Verification items for the finished model (mm, model axes). A direction names the side the tool comes from. Round coordinates to 2 decimals unless told otherwise and drop trailing zeros. Write each loop counter-clockwise with the first axis right and the second up, starting at its lowest first coordinate (ties: lowest second). Pieces come first, ordered by that corner, then holes.
Autodesk Fusion 360 part; units mm, degrees
sketch "Sketch1" plane through (0, 0, 0) normal (0, 1, 0) x (1, 0, 0)
  line L0 (0, 0) -> (49, 0)
  line L1 (49, 0) -> (49, -24)
  line L2 (49, -24) -> (0, -24)
  line L3 (0, -24) -> (0, 0)
extrude "Extrude1" add sketch "Sketch1" along normal blind 2
sketch "Sketch2" plane through (0, 0, 0) normal (0, 1, 0) x (1, 0, 0)
  line L0 (10, 0) -> (39, 0)
  line L1 (39, 0) -> (39, -14)
  line L2 (39, -14) -> (10, -14)
  line L3 (10, -14) -> (10, 0)
extrude "Extrude2" add sketch "Sketch2" against normal blind 5
fillet "Fillet1" radius 3 1 edges at (0, 1, 24)
fillet "Fillet2" radius 3 1 edges at (49, 1, 24)
fillet "Fillet3" radius 3 1 edges at (49, 1, 0)
fillet "Fillet4" radius 3 1 edges at (0, 1, 0)
sketch "Sketch3" plane through (0, 0, 0) normal (0, 1, 0) x (1, 0, 0)
  circle A0 centre (5, -5) radius 2.5
  dimension "d13" = 5
extrude "Extrude3" cut sketch "Sketch3" along normal blind 3
sketch "Sketch4" plane through (0, 0, 0) normal (0, 1, 0) x (1, 0, 0)
  circle A0 centre (44, -5) radius 2.5
  dimension "d16" = 5
extrude "Extrude4" cut sketch "Sketch4" along normal blind 3
sketch "Sketch5" plane through (0, 0, 0) normal (0, 1, 0) x (1, 0, 0)
  circle A0 centre (5, -19) radius 2.5
  dimension "d19" = 5
extrude "Extrude5" cut sketch "Sketch5" along normal blind 3
sketch "Sketch6" plane through (0, 0, 0) normal (0, 1, 0) x (1, 0, 0)
  circle A0 centre (44, -19) radius 2.5
  dimension "d22" = 5
extrude "Extrude6" cut sketch "Sketch6" along normal blind 3
sketch "Sketch7" plane through (0, 0, 0) normal (0, 1, 0) x (1, 0, 0)
  circle A0 centre (44, -12) radius 2.5
  dimension "d25" = 5
extrude "Extrude7" cut sketch "Sketch7" along normal blind 2
sketch "Sketch8" plane through (0, 0, 0) normal (0, 1, 0) x (1, 0, 0)
  circle A0 centre (5, -12) radius 2.5
  dimension "d28" = 5
extrude "Extrude8" cut sketch "Sketch8" along normal blind 3
sketch "Sketch9" plane through (0, 0, 0) normal (0, 1, 0) x (1, 0, 0)
  circle A0 centre (25, -19) radius 2.5
  dimension "d31" = 5
extrude "Extrude9" cut sketch "Sketch9" along normal blind 3
sketch "Sketch10" plane through (0, 0, 0) normal (0, 1, 0) x (1, 0, 0)
  circle A0 centre (15, -19) radius 2.5
  dimension "d34" = 5
extrude "Extrude10" cut sketch "Sketch10" along normal blind 2
sketch "Sketch11" plane through (0, 0, 0) normal (0, 1, 0) x (1, 0, 0)
  circle A0 centre (35, -19) radius 2.5
  dimension "d37" = 5
extrude "Extrude11" cut sketch "Sketch11" along normal blind 5
Q1. Release check for a two-part mould opening along Z. For faces 1 (the cylindrical face through (48.1, 1.01, 23.14)), 2 (the flat face through (24.2, 0, 14.5)), 3 (the cylindrical face through (6.34, 0.99, 21.11)) record: released by +Z, released by -Z, zero draft, split by the parting line, or undercut.
Recorded:
face 1: released by +Z
face 2: zero draft
face 3: undercut
Q2. Depth check by flat-ended pin: P1, Ø3, axis at x = 15, z = 19, coming from the -Y side; P2, Ø8, axis at x = 44, z = 5, coming from the -Y side; P3, Ø2.5, axis at x = 26.5, y = -2.5, coming from the +Z side; P4, Ø1.5, axis at y = -2.5, z = 8.5, coming from the -X side. Enter the tip coordinate at first touch or a pass-through.
Recorded:
P1: passes through
P2: stops at y = 0
P3: stops at z = 14
P4: stops at x = 10
Q3. Sectioned sample at D-D (z = 19). Enter the section's corners in (x, y), plus the area to 3 significant figures.
Recorded:
outline: (0, 0) - (2.5, 0) - (2.5, 2) - (0, 2) - close; (7.5, 0) - (12.5, 0) - (12.5, 2) - (7.5, 2) - close; (17.5, 0) - (22.5, 0) - (22.5, 2) - (17.5, 2) - close; (27.5, 0) - (32.5, 0) - (32.5, 2) - (27.5, 2) - close; (37.5, 0) - (41.5, 0) - (41.5, 2) - (37.5, 2) - close; (46.5, 0) - (49, 0) - (49, 2) - (46.5, 2) - close
area: 48.0 mm2
Q4. Sectioned sample at A-A (x = 33). Enter the section's corners in (y, z).
Recorded:
outline: (-5, 0) - (2, 0) - (2, 17.5) - (0, 17.5) - (0, 14) - (-5, 14) - close; (0, 20.5) - (2, 20.5) - (2, 24) - (0, 24) - close
Q5. Material ranges on line 1 along X through (y, z) = (0.8, 5); line 2 along X through (y, z) = (1.15, 19); line 3 along Z through (x, y) = (5, 1.4), recorded low to high.
Recorded:
line 1: x = 0 to 2.5, 7.5 to 41.5, 46.5 to 49
line 2: x = 0 to 2.5, 7.5 to 12.5, 17.5 to 22.5, 27.5 to 32.5, 37.5 to 41.5, 46.5 to 49
line 3: z = 0 to 2.5, 7.5 to 9.5, 14.5 to 16.5, 21.5 to 24
Q6. Sectioned sample at C-C (y = 1). Give the number of separate pieces and of enclosed holes in the cut face, plus the area to 3 significant figures.
Recorded:
separate pieces: 1
enclosed holes: 9
area: 992 mm2
Q7. Tool access check on faces 4 (the flat face through (39, -2, 7)), 5 (the flat face through (25, -2, 14)), 6 (the flat face through (10, -2, 7)), 7 (the flat face through (0, 1, 12)), 8 (the cylindrical face through (7.385, 0.986, 5.751)). Record the directions out of +Z, -Z, +X, -X, +Y, -Y that give a thin tool (end or side, any length) a straight path to the whole face; none if there is none.
Recorded:
face 4: +Z, -Z, +X, -Y
face 5: +Z, +X, -X, -Y
face 6: +Z, -Z, -X, -Y
face 7: +Z, -Z, -X, +Y, -Y
face 8: +Y, -Y
Q8. Sectioned sample at B-B (x = 5). Enter the section's corners in (y, z), plus the area to 3 significant figures.
Recorded:
outline: (0, 0) - (2, 0) - (2, 2.5) - (0, 2.5) - close; (0, 7.5) - (2, 7.5) - (2, 9.5) - (0, 9.5) - close; (0, 14.5) - (2, 14.5) - (2, 16.5) - (0, 16.5) - close; (0, 21.5) - (2, 21.5) - (2, 24) - (0, 24) - close
area: 18.0 mm2
